Verification items for the finished model (mm, model axes). Face numbers are marked on the shaded views. A direction names the side the tool comes from. Coordinates: 2 decimals unless noted, no trailing zeros. Loops run counter-clockwise (first coordinate to the right, second up) from the corner with the lowest first, then second, coordinate; pieces in that order, holes last. Notation, with made-up numbers: (36, 6) - (76, 6) arc R29 ccw to (76, 33) - close; hole circle Ø11 at (-32, -37). An arc over 180 degrees is marked (long way). One line per item, written item: value. Start each with the question number.
(1) Thickness scan on probe 1 along Z at (x, y) = (39.5, 2); probe 2 along X at (y, z) = (1.55, -3.1); probe 3 along Z at (x, y) = (2.85, 1.5). Record the ranges inside material, lowest first. Write a range as [from, to].
(2) Section check B-B (z = -18.5). Record the boundary of the cut face in (x, y).
(3) Section check A-A (x = 2.85). Record the boundary of the cut face in (y, z).
(4) Section check D-D (x = 16). Record the boundary of the cut face in (y, z), plus the area to 3 significant figures.
(5) Set-up check for the marked faces 4 and 5: record each of +Z, -Z, +X, -X, +Y, -Y from which the full face is reachable in a straight line by a thin tool's end or side.
(6) Draft check along X on the marked faces 1, 2 and 3. Enter one of: +X half, -X half, draft (parallel to the pull), parting line (faces both ways), or undercut.
(7) Gauge pin test, flat end, axial feed: P1, Ø5, axis at x = 39.5, z = -21, coming from the +Y side. Record the tip position at first contact, or that the pin passes through.
(8) Section check C-C (y = 1.95). Record the boundary of the cut face in (x, z), plus the area to 3 significant figures.
```python
from build123d import *

# Parameters (mm, degrees)
SKETCH1_W           = 42.5
SKETCH1_H           = 24
SKETCH1_R           = 1.35
SKETCH1_R_2         = 1.5
BOSS_EXTRUDE1_DEPTH = 3
SKETCH2_W           = 0.15
SKETCH2_H           = 3
CUT_EXTRUDE1_DEPTH  = 4
FILLET1_R           = 2


with BuildPart() as part:
    # Sketch1 → Boss-Extrude1 (new body)
    with BuildSketch(Plane(origin=(0, 0, 0), x_dir=(1, 0, 0), z_dir=(0, 1, 0))):
        with Locations((21.25, 12)):
            Rectangle(SKETCH1_W, SKETCH1_H)
        with Locations((2.85, 3.1)):
            Circle(SKETCH1_R, mode=Mode.SUBTRACT)
        with Locations((29.95, 3.1)):
            Circle(SKETCH1_R, mode=Mode.SUBTRACT)
        with Locations((39.5, 3)):
            Circle(SKETCH1_R_2, mode=Mode.SUBTRACT)
        Polygon((5, 6), (5, 18), (10.5, 18), (10.5, 21), (22.5, 21), (22.5, 18), (28, 18), (28, 6), (22.5, 6), (22.5, 3), (10.5, 3), (10.5, 6), align=None, mode=Mode.SUBTRACT)
        with Locations((2.85, 20.9)):
            Circle(SKETCH1_R, mode=Mode.SUBTRACT)
        with Locations((29.95, 20.9)):
            Circle(SKETCH1_R, mode=Mode.SUBTRACT)
        with Locations((39.5, 21)):
            Circle(SKETCH1_R_2, mode=Mode.SUBTRACT)
    extrude(amount=BOSS_EXTRUDE1_DEPTH)

    # Sketch2 → Cut-Extrude1 (cut, through all)
    with BuildSketch(Plane(origin=(0, 3, 0), x_dir=(1, 0, 0), z_dir=(0, 1, 0))):
        with Locations((22.575, 4.5)):
            Rectangle(SKETCH2_W, SKETCH2_H)
        with Locations((10.425, 4.5)):
            Rectangle(SKETCH2_W, SKETCH2_H)
        with Locations((22.575, 19.5)):
            Rectangle(SKETCH2_W, SKETCH2_H)
        with Locations((10.425, 19.5)):
            Rectangle(SKETCH2_W, SKETCH2_H)
    extrude(amount=-CUT_EXTRUDE1_DEPTH, mode=Mode.SUBTRACT)

    # Fillet1
    fillet1_edges = [part.edges().sort_by_distance(p)[0] for p in [
        (0, 1.5, 0),
        (0, 1.5, -24),
        (42.5, 1.5, -24),
        (42.5, 1.5, 0),
    ]]
    fillet(fillet1_edges, radius=FILLET1_R)


solid = part.part
```
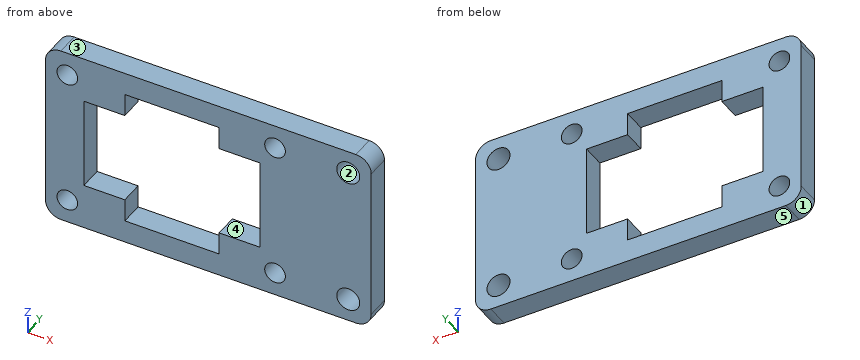
Responses:
1. probe 1: z = [-24, -22.5], [-19.5, -4.5], [-1.5, 0]
1. probe 2: x = [0, 1.5], [4.2, 10.35], [22.65, 28.6], [31.3, 38], [41, 42.5]
1. probe 3: z = [-24, -22.25], [-19.55, -4.45], [-1.75, 0]
2. outline: (0, 0) - (10.35, 0) - (10.35, 3) - (0, 3) - close; (22.65, 0) - (42.5, 0) - (42.5, 3) - (22.65, 3) - close
3. outline: (0, -24) - (3, -24) - (3, -22.25) - (0, -22.25) - close; (0, -19.55) - (3, -19.55) - (3, -4.45) - (0, -4.45) - close; (0, -1.75) - (3, -1.75) - (3, 0) - (0, 0) - close
4. outline: (0, -24) - (3, -24) - (3, -21) - (0, -21) - close; (0, -3) - (3, -3) - (3, 0) - (0, 0) - close
4. area: 18.0 mm²
5. face 4: +Y, -Y
5. face 5: -Z, +X, -X, +Y, -Y
6. face 1: -X half
6. face 2: undercut
6. face 3: draft
7. P1: stops at y = 3
8. outline: (0, -22) arc R2 ccw to (2, -24) - (40.5, -24) arc R2 ccw to (42.5, -22) - (42.5, -2) arc R2 ccw to (40.5, 0) - (2, 0) arc R2 ccw to (0, -2) - close; hole circle Ø2.7 at (2.85, -20.9); hole circle Ø2.7 at (2.85, -3.1); hole (5, -18) - (10.35, -18) - (10.35, -21) - (22.65, -21) - (22.65, -18) - (28, -18) - (28, -6) - (22.65, -6) - (22.65, -3) - (10.35, -3) - (10.35, -6) - (5, -6) - close; hole circle Ø2.7 at (29.95, -20.9); hole circle Ø2.7 at (29.95, -3.1); hole circle Ø3 at (39.5, -21); hole circle Ø3 at (39.5, -3)
8. area: 630 mm²
